Autodesk Inventor part; units mm, degrees
ref_plane "YZ Plane" through (0, 0, 0) normal (1, 0, 0) x (0, 1, 0)
ref_plane "XZ Plane" through (0, 0, 0) normal (0, 1, 0) x (-1, 0, 0)
ref_plane "XY Plane" through (0, 0, 0) normal (0, 0, 1) x (1, 0, 0)
sketch "Sketch1" plane through (0, 0, 0) normal (0, 0, 1) x (1, 0, 0)
  line L0 (-3, 22.15) -> (-3, 34.65)
  line L1 (-3, 17.15) -> (-3, 22.15)
  line L2 (-3, -3.35) -> (-3, 17.15)
  line L3 (0, -3.35) -> (-3, -3.35)
  line L4 (0, 17.15) -> (0, -3.35)
  line L5 (0, 17.15) -> (-3, 17.15)
  line L6 (-3, 34.65) -> (-3, 39.65)
  line L7 (-3, -3.35) -> (-22, -3.35)
  line L8 (-22, -3.35) -> (-22, 39.65)
  line L9 (-22, 39.65) -> (-3, 39.65)
  line L10 (-22, 39.65) -> (-25, 39.65)
  line L11 (-25, 39.65) -> (-25, 34.65)
  line L12 (-25, 34.65) -> (-22, 34.65)
  line L13 (-22, 34.65) -> (-22, 39.65)
  line L14 (-22, 24.65) -> (-11.5, 24.65)
  line L15 (-11.5, 24.65) -> (-11.5, 14.65)
  line L16 (-11.5, 14.65) -> (-22, 14.65)
  line L17 (-22, 14.65) -> (-25, 14.65)
  line L18 (-25, 14.65) -> (-25, 9.65)
  line L19 (-25, 9.65) -> (-22, 9.65)
  line L20 (-22, 9.65) -> (-22, 14.65)
  line L21 (-22, -3.35) -> (-25, -3.35)
  line L22 (-25, -3.35) -> (-25, 1.65)
  line L23 (-25, 1.65) -> (-22, 1.65)
  line L24 (-22, 1.65) -> (-22, -3.35)
  line L25 (-15, -3.35) -> (-10, -3.35)
  line L26 (-10, -3.35) -> (-10, -0.35)
  line L27 (-10, -0.35) -> (-15, -0.35)
  line L28 (-15, -0.35) -> (-15, -3.35)
  line L29 (-3, 22.15) -> (-3, 34.65)
  line L30 (0, 22.15) -> (-3, 22.15)
  line L31 (0, 34.65) -> (0, 22.15)
  line L32 (0, 34.65) -> (-3, 34.65)
  point P0 (-11.5, 19.65)
  point P1 (-3, 19.65)
  point P2 (-12.5, -3.35)
  dimension "d1" = 19
  dimension "d2" = 3
  dimension "d3" = 5
  dimension "d4" = 10
  dimension "d8" = 3
  dimension "d9" = 5
  dimension "d10" = 3
  dimension "d11" = 5
  dimension "d12" = 5
  dimension "d13" = 3
  dimension "d16" = 8.5
extrude "Extrusion1" add sketch "Sketch1" along normal blind 3 contours L1 L2 L7 L26 L27 L28 L8 L16 L15 L14 L9 L6 L0 | L0 L32 L31 L30 | L5 L4 L3 L2 | L8 L12 L11 L10 | L21 L22 L23 L8 | L8 L19 L18 L17
properties part number "SideLeftTopNM" material "Acrylic, Clear"
For this review, take the finished solid that the model builds, in its own axes (mm). A direction names the side the tool comes from. Round coordinates to 2 decimals unless told otherwise and drop trailing zeros. Write each loop counter-clockwise with the first axis right and the second up, starting at its lowest first coordinate (ties: lowest second). Pieces come first, ordered by that corner, then holes. Notation, with made-up numbers: (75.25, -13) -> (115.25, -13) arc R24 ccw to (115.25, 8) -> close; hole circle Ø5 at (-9, 29.5). An arc over 180 degrees is marked (long way). Use one line per item in the form item = value.
1) Mouldability with a two-part tool opening along X and no side actions: class faces 1 (the flat face through (-12, -0.35, 1)), 2 (the flat face through (-10, 18, 0)), 3 (the flat face through (-3, 37, 1)), 4 (the flat face through (-22, 30, 1)) as +X half, -X half, draft (parallel to the pull), parting line (faces both ways), or undercut.
Found:
face_1 = undercut
face_2 = draft
face_3 = +X half
face_4 = -X half
2) Take a section at D-D, the plane y = 19. Write out the cut boundary in (x, z), and give its area (3 significant figures).
Found:
outline = (-11.5, 0) -> (-3, 0) -> (-3, 3) -> (-11.5, 3) -> close
area = 25.5 mm2
3) Tool access review of faces 5 (the flat face through (-15, -2, 1)), 6 (the flat face through (-14, 39.65, 1)), 7 (the flat face through (-24, 34.65, 1)), 8 (the flat face through (-1, 17.15, 1)), 9 (the flat face through (-1, 34.65, 1)): name each direction out of +Z, -Z, +X, -X, +Y, -Y from which nothing blocks a thin tool from reaching the whole face with its end or side.
Found:
face_5 = +Z, -Z, -Y
face_6 = +Z, -Z, +X, -X, +Y
face_7 = +Z, -Z, -X
face_8 = +Z, -Z, +X
face_9 = +Z, -Z, +X, +Y
4) To check wall thickness, follow L1, parallel to Y at x = -23.5, z = 2; L2, parallel to Y at x = -18.75, z = 1.85; L3, parallel to Y at x = -1.5, z = 2.55. State the ranges of each line that lie inside material, in increasing order. Write a range as from..to.
Found:
L1 = -3.35..1.65, 9.65..14.65, 34.65..39.65
L2 = -3.35..14.65, 24.65..39.65
L3 = -3.35..17.15, 22.15..34.65
5) Take a section at C-C, the plane z = 2.1. Write out the cut boundary in (x, y), and give its area (3 significant figures).
Found:
outline = (-25, -3.35) -> (-15, -3.35) -> (-15, -0.35) -> (-10, -0.35) -> (-10, -3.35) -> (0, -3.35) -> (0, 17.15) -> (-3, 17.15) -> (-3, 22.15) -> (0, 22.15) -> (0, 34.65) -> (-3, 34.65) -> (-3, 39.65) -> (-25, 39.65) -> (-25, 34.65) -> (-22, 34.65) -> (-22, 24.65) -> (-11.5, 24.65) -> (-11.5, 14.65) -> (-25, 14.65) -> (-25, 9.65) -> (-22, 9.65) -> (-22, 1.65) -> (-25, 1.65) -> close
area = 841 mm2
6) Take a section at A-A, the plane x = -13.5. Write out the cut boundary in (y, z), and give its area (3 significant figures).
Found:
outline = (-0.35, 0) -> (14.65, 0) -> (14.65, 3) -> (-0.35, 3) -> close; (24.65, 0) -> (39.65, 0) -> (39.65, 3) -> (24.65, 3) -> close
area = 90.0 mm2
7) Clearance check with flat-ended pins moving along their axes: pin 1 (0.9 mm diameter, centred on y = 32, z = 1.5, fed in from -X); pin 2 (0.9 mm diameter, centred on x = -12.5, z = 1.5, fed in from -Y); pin 3 (0.9 mm diameter, centred on x = -1, z = 1.5, fed in from +Y). State where each tip first meets the part, or that it passes through.
Found:
pin_1 = -22
pin_2 = -0.35
pin_3 = 34.65
8) Take a section at B-B, the plane x = -23. Write out the cut boundary in (y, z), and give its area (3 significant figures).
Found:
outline = (-3.35, 0) -> (1.65, 0) -> (1.65, 3) -> (-3.35, 3) -> close; (9.65, 0) -> (14.65, 0) -> (14.65, 3) -> (9.65, 3) -> close; (34.65, 0) -> (39.65, 0) -> (39.65, 3) -> (34.65, 3) -> close
area = 45.0 mm2
